Design review of the part built by this model. Coordinates are the model's own, in mm. A direction names the side the tool comes from. Give positions to 0.01 mm unless a question says otherwise; leave off trailing zeros. Loops run counter-clockwise (first coordinate to the right, second up) from the corner with the lowest first, then second, coordinate; pieces in that order, holes last. Notation, with made-up numbers: (66, 0.25) -> (116, 0.25) arc R11 cw to (116, 9.25) -> close; hole circle Ø1 at (-9, -6.5). An arc over 180 degrees is marked (long way). Answer in a Markdown table with one row per item. Add a question column.
(1) Consider section C-C on x = 321. Write out the cut boundary in (y, z), then the cut area to 3 significant figures.
(2) Consider section A-A on y = 0. Write out the cut boundary in (x, z).
(3) Consider section B-B on z = 8.5. Write out the cut boundary in (x, y), then the cut area to 3 significant figures.
(4) For faces 1 (the flat face through (215.112, -59.403, 24.65)), 2 (the cylindrical face through (-2.17, -9.76, 40.14)), list the 3-axis set-ups (+Z, -Z, +X, -X, +Y, -Y) from which the entire face can be reached by the end or side of a thin tool; tool diameter is ignored.
(5) Consider section D-D on x = 160.5. Write out the cut boundary in (y, z).
(6) Draft analysis for pull direction X (two halves, no side actions). For faces 3 (the cylindrical face through (-79.98, -1.76, 24.65)), 4 (the cylindrical face through (359.992, 0.78, 24.65)), 5 (the flat face through (0, 0, 30)), state which applies: +X half, -X half, draft (parallel to the pull), parting line (faces both ways), or undercut.
(7) For pin 1 (12 mm diameter, centred on x = 320, y = 0, fed in from -Z); pin 2 (4 mm diameter, centred on y = -39, z = 9, fed in from +X); pin 3 (1.5 mm diameter, centred on y = 39.5, z = 39.5, fed in from -X); pin 4 (10 mm diameter, centred on x = 322, y = 2.5, fed in from +Z), all flat-tipped, find the tip position at first contact; note any pin that passes through.
(8) For line 1 (Y direction, x = 0, z = 34.5); line 2 (X direction, y = -4.5, z = 42); line 3 (Y direction, x = 320, z = 42), list the stretches that pass through material, from the lowest coordinate up.
from build123d import *

# Parameters (mm, degrees)
BOSS_EXTRUDE1_DEPTH = 50
SKETCH2_R           = 10
CUT_EXTRUDE1_DEPTH  = 20


with BuildPart() as part:
    # Sketch1 → Boss-Extrude1 (new body)
    with BuildSketch(Plane.XY):
        with BuildLine():
            Line((0, 80), (100, 80))
            Line((100, 80), (327.045328578, 39.374653589))
            ThreePointArc((327.045328578, 39.374653589), (360, 0), (327.045328578, -39.374653589))
            Line((327.045328578, -39.374653589), (100, -80))
            Line((100, -80), (0, -80))
            ThreePointArc((0, -80), (-80, 0), (0, 80))
        make_face()
    extrude(amount=BOSS_EXTRUDE1_DEPTH)

    # Sketch2 → Cut-Extrude1 (cut)
    with BuildSketch(Plane.XY.offset(50)):
        Circle(SKETCH2_R)
        with Locations((320, 0)):
            Circle(SKETCH2_R)
    extrude(amount=-CUT_EXTRUDE1_DEPTH, mode=Mode.SUBTRACT)


solid = part.part
Values follow:
| question | item | result |
|---|---|---|
| 1 | outline | (-40.46, 0) -> (40.46, 0) -> (40.46, 50) -> (9.95, 50) -> (9.95, 30) -> (-9.95, 30) -> (-9.95, 50) -> (-40.46, 50) -> close |
| 1 | area | 3,650 mm2 |
| 2 | outline | (-80, 0) -> (360, 0) -> (360, 50) -> (330, 50) -> (330, 30) -> (310, 30) -> (310, 50) -> (10, 50) -> (10, 30) -> (-10, 30) -> (-10, 50) -> (-80, 50) -> close |
| 3 | outline | (0, -80) -> (100, -80) -> (327.05, -39.37) arc R40 ccw to (327.05, 39.37) -> (100, 80) -> (0, 80) arc R80 ccw to start |
| 3 | area | 55,100 mm2 |
| 4 | face 1 | +Z, -Z, +X, -Y |
| 4 | face 2 | +Z |
| 5 | outline | (-69.17, 0) -> (69.17, 0) -> (69.17, 50) -> (-69.17, 50) -> close |
| 6 | face 3 | -X half |
| 6 | face 4 | +X half |
| 6 | face 5 | undercut |
| 7 | pin 1 | z = 0 |
| 7 | pin 2 | x = 335.2 |
| 7 | pin 3 | x = -69.99 |
| 7 | pin 4 | z = 30 |
| 8 | line 1 | -80 to -10, 10 to 80 |
| 8 | line 2 | -79.87 to -8.93, 8.93 to 311.07, 328.93 to 359.75 |
| 8 | line 3 | -40.64 to -10, 10 to 40.64 |
